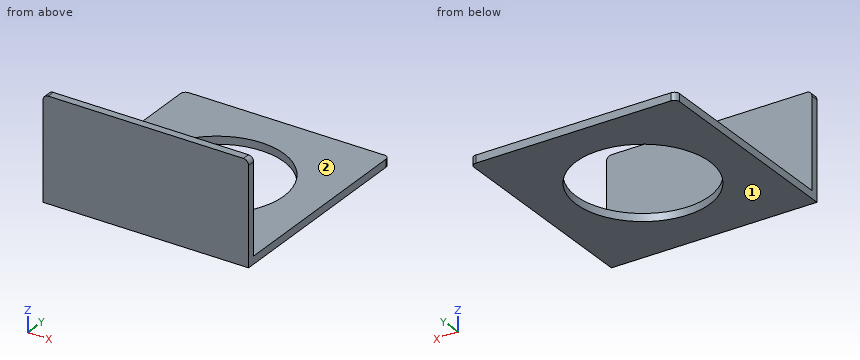
```python
from build123d import *

# Parameters (mm, degrees)
SKETCH1_W           = 40
SKETCH1_H           = 41.5
BOSS_EXTRUDE1_DEPTH = 1.5
SKETCH2_W           = 40
SKETCH2_H           = 1.5
BOSS_EXTRUDE2_DEPTH = 18.5
FILLET1_R           = 1
FILLET2_R           = 1
SKETCH3_R           = 13
CUT_EXTRUDE1_DEPTH  = 1.5


with BuildPart() as part:
    # Sketch1 → Boss-Extrude1 (new body)
    with BuildSketch(Plane.XY):
        with Locations((20, 20.75)):
            Rectangle(SKETCH1_W, SKETCH1_H)
    extrude(amount=BOSS_EXTRUDE1_DEPTH)

    # Sketch2 → Boss-Extrude2 (add)
    with BuildSketch(Plane.XY.offset(1.5)):
        with Locations((20, 0.75)):
            Rectangle(SKETCH2_W, SKETCH2_H)
    extrude(amount=BOSS_EXTRUDE2_DEPTH)

    # Fillet1
    fillet1_edges = [part.edges().sort_by_distance(p)[0] for p in [
        (0, 41.5, 0.75),
    ]]
    fillet(fillet1_edges, radius=FILLET1_R)

    # Fillet2
    fillet2_edges = [part.edges().sort_by_distance(p)[0] for p in [
        (0, 0.75, 20),
        (40, 0.75, 20),
        (40, 41.5, 0.75),
    ]]
    fillet(fillet2_edges, radius=FILLET2_R)

    # Sketch3 → Cut-Extrude1 (cut)
    with BuildSketch(Plane.XY.offset(1.5)):
        with Locations((20, 21)):
            Circle(SKETCH3_R)
    extrude(amount=-CUT_EXTRUDE1_DEPTH, mode=Mode.SUBTRACT)


solid = part.part
```
Source: CAD feature listing. Evaluate the final solid. Frame: model axes, mm. Face numbers are marked on the shaded views. A direction names the side the tool comes from. Coordinates: 2 decimals unless noted, no trailing zeros. Loops run counter-clockwise (first coordinate to the right, second up) from the corner with the lowest first, then second, coordinate; pieces in that order, holes last. Notation, with made-up numbers: (-20, 78) -> (24, 78) arc R18 ccw to (24, 98) -> close; hole circle Ø8 at (36, -34). An arc over 180 degrees is marked (long way). One line per item, written item: value. Start each with the question number.
Q1. Section query D-D, the plane z = 16.5. Return the cut outline in (x, y).
Q2. Contact query for flat-ended pins moving along their axis: P1, Ø5, axis at x = 24, z = 15.5, coming from the -Y side; P2, Ø1, axis at x = 28, z = 9.5, coming from the +Y side. Output: stop coordinate, or through.
Q3. Set-up query: the marked faces 1 and 2. Return all of +Z, -Z, +X, -X, +Y, -Y with unobstructed straight access to the full face (end or side cutting, diameter ignored); none if empty.
Q4. Section query C-C, the plane x = 5.5. Return the cut outline in (y, z), and give its area (3 significant figures).
Q5. Line query: line 1 along Y through (x, z) = (20, 0.8); line 2 along Z through (x, y) = (21.5, 6.5). Output: solid intervals per line, ascending.
Q6. Section query B-B, the plane y = 21. Return the cut outline in (x, z), and give its area (3 significant figures).
Q7. Section query A-A, the plane x = 20. Return the cut outline in (y, z).
Results:
1. outline: (0, 0) -> (40, 0) -> (40, 1.5) -> (0, 1.5) -> close
2. P1: y = 0
2. P2: y = 1.5
3. face 1: -Z, +X, -X, +Y, -Y
3. face 2: +Z, +X, -X, +Y
4. outline: (0, 0) -> (41.5, 0) -> (41.5, 1.5) -> (1.5, 1.5) -> (1.5, 20) -> (0, 20) -> close
4. area: 90.0 mm^2
5. line 1: 0 to 8, 34 to 41.5
5. line 2: 0 to 1.5
6. outline: (0, 0) -> (7, 0) -> (7, 1.5) -> (0, 1.5) -> close; (33, 0) -> (40, 0) -> (40, 1.5) -> (33, 1.5) -> close
6. area: 21.0 mm^2
7. outline: (0, 0) -> (8, 0) -> (8, 1.5) -> (1.5, 1.5) -> (1.5, 20) -> (0, 20) -> close; (34, 0) -> (41.5, 0) -> (41.5, 1.5) -> (34, 1.5) -> close
